Here's how the part is built. I have some questions about the finished solid (model axes, mm). Face numbers are marked on the shaded views. A direction names the side the tool comes from. Round coordinates to 2 decimals unless told otherwise and drop trailing zeros. Write each loop counter-clockwise with the first axis right and the second up, starting at its lowest first coordinate (ties: lowest second). Pieces come first, ordered by that corner, then holes. Notation, with made-up numbers: (48.5, 60.5) -> (105.5, 60.5) arc R20 ccw to (105.5, 72.5) -> close; hole circle Ø6 at (-33, 41). An arc over 180 degrees is marked (long way). Answer as CSV lines item,"result".
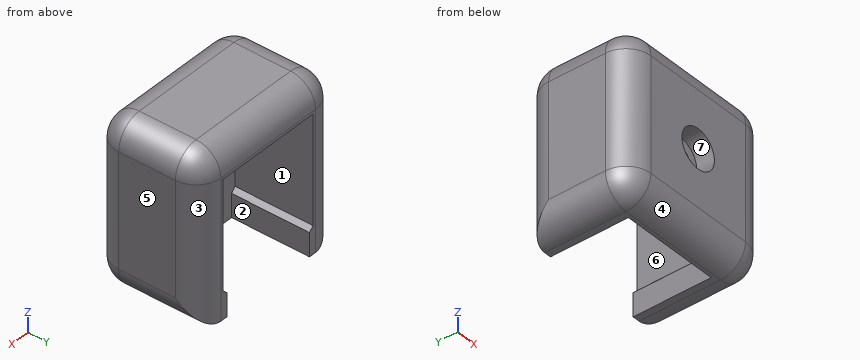
```python
from build123d import *

# Parameters (mm, degrees)
SKETCH_1_W                   = 46
SKETCH_1_H                   = 46
EXTRUDE_1_DEPTH              = 30
SKETCH_2_W                   = 30.4
SKETCH_2_H                   = 30.4
CUT_EXTRUDE_1_DEPTH          = 22
SKETCH_3_W                   = 28
SKETCH_3_H                   = 7.8
CUT_EXTRUDE_2_DEPTH          = 22
FILLET_1_R                   = 7
HOLE_WIZARD_M6_1_D           = 6.2
HOLE_WIZARD_M6_1_CBORE_D     = 11
HOLE_WIZARD_M6_1_CBORE_DEPTH = 5
CHAMFER_1_SIZE               = 1.2


with BuildPart() as part:
    # 草图1 → 凸台-拉伸1 (new body)
    with BuildSketch(Plane(origin=(0, 0, 0), x_dir=(1, 0, 0), z_dir=(0, 1, 0))):
        Rectangle(SKETCH_1_W, SKETCH_1_H)
    extrude(amount=EXTRUDE_1_DEPTH)

    # 草图2 → 切除-拉伸1 (cut)
    with BuildSketch(Plane(origin=(0, 30, 0), x_dir=(1, 0, 0), z_dir=(0, 1, 0))):
        Rectangle(SKETCH_2_W, SKETCH_2_H)
    extrude(amount=-CUT_EXTRUDE_1_DEPTH, mode=Mode.SUBTRACT)

    # 草图3 → 切除-拉伸2 (cut)
    with BuildSketch(Plane(origin=(0, 30, 0), x_dir=(1, 0, 0), z_dir=(0, 1, 0))):
        with Locations((0, 19.1)):
            Rectangle(SKETCH_3_W, SKETCH_3_H)
    extrude(amount=-CUT_EXTRUDE_2_DEPTH, mode=Mode.SUBTRACT)

    # 圆角1
    fillet_1_edges = [part.edges().sort_by_distance(p)[0] for p in [
        (-23, 30, 0),
        (0, 30, 23),
        (23, 30, 0),
        (0, 0, 23),
        (-23, 0, 0),
        (0, 0, -23),
        (23, 0, 0),
        (23, 15, 23),
        (-23, 15, 23),
        (-23, 15, -23),
        (23, 15, -23),
    ]]
    fillet(fillet_1_edges, radius=FILLET_1_R)

    # M6 六角头螺钉的柱形沉头孔1 (through all)
    with Locations(Plane(origin=(0, 0, 0), x_dir=(-1, 0, 0), z_dir=(0, -1, 0))):
        with Locations((0, 0)):
            CounterBoreHole(HOLE_WIZARD_M6_1_D / 2, HOLE_WIZARD_M6_1_CBORE_D / 2, HOLE_WIZARD_M6_1_CBORE_DEPTH)

    # 倒角1
    chamfer_1_edges = [part.edges().sort_by_distance(p)[0] for p in [
        (14, 19, -15.2),
        (-14, 19, -15.2),
    ]]
    chamfer(chamfer_1_edges, length=CHAMFER_1_SIZE - 0.0001)  # a hair under: the kernel refuses the full size


solid = part.part
```
1. If I drill on line 1 (Z direction, x = 0, y = 6.85); line 2 (X direction, y = 19.5, z = 7); line 3 (Y direction, x = -13, z = -5), over which ranges is the centre line in solid material (lowest first)?
Numbers:
line 1,"z = -23 to -3.1, 3.1 to 23"
line 2,"x = -23 to -15.2, 15.2 to 23"
line 3,"y = 0 to 8"
2. If we mould it in two halves opening along Z, with no side actions, what happens to the marked faces 4, 5, 6 and 7? For each: released by +Z, released by -Z, zero draft, split by the parting line, or undercut.
Numbers:
face 4,"released by -Z"
face 5,"zero draft"
face 6,"undercut"
face 7,"undercut"
3. On a 3-axis mill with a long thin cutter (end or side, diameter ignored), from which of +Z, -Z, +X, -X, +Y, -Y can I reach the whole of each face in a straight line? I mean the marked faces 1, 2 and 3. Say none if no direction works.
Numbers:
face 1,"+Y"
face 2,"-Z, +Y"
face 3,"+Z, -Z, +X, +Y"
4. Suppose I cut it at C-C on z = -7. Please give me the cut outline in (x, y), and give its area (3 significant figures).
Numbers:
outline,"(-23, 7) arc R7 ccw to (-16, 0) -> (16, 0) arc R7 ccw to (23, 7) -> (23, 23) arc R7 ccw to (16, 30) -> (15.2, 30) -> (15.2, 8) -> (-15.2, 8) -> (-15.2, 30) -> (-16, 30) arc R7 ccw to (-23, 23) -> close"
area,"669 mm^2"
5. Suppose I cut it at A-A on z = 0. Please give me the cut outline in (x, y).
Numbers:
outline,"(-23, 7) arc R7 ccw to (-16, 0) -> (-5.5, 0) -> (-5.5, 5) -> (-3.1, 5) -> (-3.1, 8) -> (-15.2, 8) -> (-15.2, 30) -> (-16, 30) arc R7 ccw to (-23, 23) -> close; (3.1, 5) -> (5.5, 5) -> (5.5, 0) -> (16, 0) arc R7 ccw to (23, 7) -> (23, 23) arc R7 ccw to (16, 30) -> (15.2, 30) -> (15.2, 8) -> (3.1, 8) -> close"
6. Suppose I cut it at B-B on x = 0. Please give me the cut outline in (y, z), and give its area (3 significant figures).
Numbers:
outline,"(0, -16) arc R7 ccw to (7, -23) -> (8, -23) -> (8, -3.1) -> (5, -3.1) -> (5, -5.5) -> (0, -5.5) -> close; (0, 5.5) -> (5, 5.5) -> (5, 3.1) -> (8, 3.1) -> (8, 15.2) -> (30, 15.2) -> (30, 16) arc R7 ccw to (23, 23) -> (7, 23) arc R7 ccw to (0, 16) -> close"
area,"434 mm^2"
7. For pin 1 Ø6.5 at (x, z) = (0, 0) entering from -Y; pin 2 Ø6.5 at (x, y) = (3.5, 17) entering from -Z; pin 3 Ø8 at (x, z) = (5.5, 4) entering from +Y; pin 4 Ø3.5 at (x, z) = (0, 0) entering from -Y, each with a flat end and sliding along its axis, tell me the tip position at first contact or that it passes through.
Numbers:
pin 1,"stops at y = 5"
pin 2,"stops at z = 15.2"
pin 3,"stops at y = 8"
pin 4,"passes through"
